```python
from build123d import *

# Parameters (mm, degrees)
SKETCH1_R           = 3.175
BOSS_EXTRUDE1_DEPTH = 3.175
SKETCH2_R           = 3.2004
SKETCH2_R_2         = 2.4384
SKETCH2_R_3         = 3.175
CUT_EXTRUDE2_DEPTH  = 205.115710138
SKETCH3_R           = 4.73075
CUT_EXTRUDE3_DEPTH  = 1.5875
CUT_EXTRUDE4_DEPTH  = 205.115710138


with BuildPart() as part:
    # Sketch1 → Boss-Extrude1 (new body)
    with BuildSketch(Plane(origin=(0, 0, 0), x_dir=(0, 0, -1), z_dir=(1, 0, 0))):
        with BuildLine():
            Line((12.7, 19.05), (0, 19.05))
            ThreePointArc((0, 19.05), (-19.05, 0), (0, -19.05))
            Line((0, -19.05), (12.7, -19.05))
            Line((12.7, -19.05), (12.7, -15.875))
            Line((12.7, -15.875), (25.4, -15.875))
            Line((25.4, -15.875), (25.4, -19.05))
            Line((25.4, -19.05), (38.1, -19.05))
            Line((38.1, -19.05), (38.1, -15.875))
            Line((38.1, -15.875), (50.8, -15.875))
            Line((50.8, -15.875), (50.8, -19.05))
            Line((50.8, -19.05), (63.5, -19.05))
            Line((63.5, -19.05), (63.5, -15.875))
            Line((63.5, -15.875), (76.2, -15.875))
            Line((76.2, -15.875), (76.2, -19.05))
            Line((76.2, -19.05), (88.9, -19.05))
            Line((88.9, -19.05), (88.9, -15.875))
            Line((88.9, -15.875), (101.6, -15.875))
            Line((101.6, -15.875), (101.6, -19.05))
            Line((101.6, -19.05), (114.3, -19.05))
            Line((114.3, -19.05), (114.3, -15.875))
            Line((114.3, -15.875), (127, -15.875))
            Line((127, -15.875), (127, -19.05))
            Line((127, -19.05), (139.7, -19.05))
            Line((139.7, -19.05), (139.7, -15.875))
            Line((139.7, -15.875), (152.4, -15.875))
            Line((152.4, -15.875), (152.4, -19.05))
            Line((152.4, -19.05), (165.1, -19.05))
            Line((165.1, -19.05), (165.1, -15.875))
            Line((165.1, -15.875), (177.8, -15.875))
            Line((177.8, -15.875), (177.8, -19.05))
            Line((177.8, -19.05), (190.5, -19.05))
            Line((190.5, -19.05), (190.5, -15.875))
            Line((190.5, -15.875), (203.2, -15.875))
            Line((203.2, -15.875), (203.2, 15.875))
            Line((203.2, 15.875), (190.5, 15.875))
            Line((190.5, 15.875), (190.5, 19.05))
            Line((190.5, 19.05), (177.8, 19.05))
            Line((177.8, 19.05), (177.8, 15.875))
            Line((177.8, 15.875), (165.1, 15.875))
            Line((165.1, 15.875), (165.1, 19.05))
            Line((165.1, 19.05), (152.4, 19.05))
            Line((152.4, 19.05), (152.4, 15.875))
            Line((152.4, 15.875), (139.7, 15.875))
            Line((139.7, 15.875), (139.7, 19.05))
            Line((139.7, 19.05), (127, 19.05))
            Line((127, 19.05), (127, 15.875))
            Line((127, 15.875), (114.3, 15.875))
            Line((114.3, 15.875), (114.3, 19.05))
            Line((114.3, 19.05), (101.6, 19.05))
            Line((101.6, 19.05), (101.6, 15.875))
            Line((101.6, 15.875), (88.9, 15.875))
            Line((88.9, 15.875), (88.9, 19.05))
            Line((88.9, 19.05), (76.2, 19.05))
            Line((76.2, 19.05), (76.2, 15.875))
            Line((76.2, 15.875), (63.5, 15.875))
            Line((63.5, 15.875), (63.5, 19.05))
            Line((63.5, 19.05), (50.8, 19.05))
            Line((50.8, 19.05), (50.8, 15.875))
            Line((50.8, 15.875), (38.1, 15.875))
            Line((38.1, 15.875), (38.1, 19.05))
            Line((38.1, 19.05), (25.4, 19.05))
            Line((25.4, 19.05), (25.4, 15.875))
            Line((25.4, 15.875), (12.7, 15.875))
            Line((12.7, 15.875), (12.7, 19.05))
        make_face()
        Circle(SKETCH1_R, mode=Mode.SUBTRACT)
    extrude(amount=BOSS_EXTRUDE1_DEPTH)

    # Sketch2 → Cut-Extrude2 (cut, through all)
    with BuildSketch(Plane(origin=(3.175, 0, 0), x_dir=(0, 0, -1), z_dir=(1, 0, 0))):
        with Locations((15.875, 0)):
            Circle(SKETCH2_R)
        with Locations((187.325, 0)):
            Circle(SKETCH2_R_2)
        with Locations((42.8625, 0)):
            Circle(SKETCH2_R_3)
        with Locations((77.7875, 0)):
            Circle(SKETCH2_R_3)
    extrude(amount=-CUT_EXTRUDE2_DEPTH, mode=Mode.SUBTRACT)

    # Sketch3 → Cut-Extrude3 (cut)
    with BuildSketch(Plane(origin=(3.175, 0, 0), x_dir=(0, 0, -1), z_dir=(1, 0, 0))):
        with Locations((15.875, 0)):
            Circle(SKETCH3_R)
        Polygon((3.229899478, -5.59435), (6.459798957, 0), (3.229899478, 5.59435), (-3.229899478, 5.59435), (-6.459798957, 0), (-3.229899478, -5.59435), align=None)
    extrude(amount=-CUT_EXTRUDE3_DEPTH, mode=Mode.SUBTRACT)

    # Sketch4 → Cut-Extrude4 (cut, through all)
    with BuildSketch(Plane(origin=(3.175, 0, 0), x_dir=(0, 0, -1), z_dir=(1, 0, 0))):
        with BuildLine():
            Line((133.35, 3.175), (158.75, 3.175))
            ThreePointArc((158.75, 3.175), (161.925, 0), (158.75, -3.175))
            Line((158.75, -3.175), (133.35, -3.175))
            ThreePointArc((133.35, -3.175), (130.175, 0), (133.35, 3.175))
        make_face()
    extrude(amount=-CUT_EXTRUDE4_DEPTH, mode=Mode.SUBTRACT)


solid = part.part
```
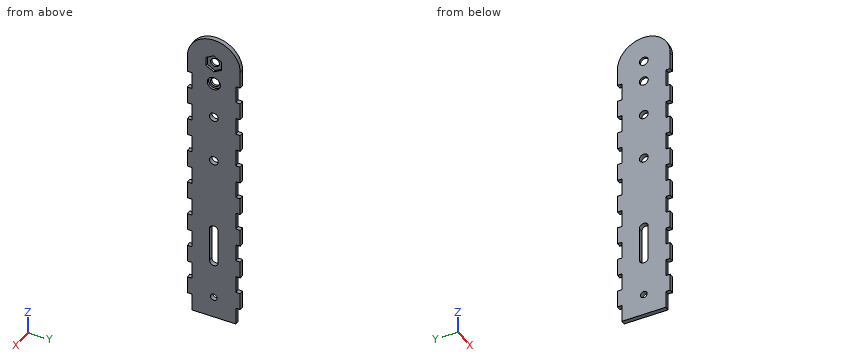
CAD build for the part. Positions are in the model's coordinates, mm. Coordinates: 2 decimals unless noted, no trailing zeros.
(1) Drill centre lines: L1, parallel to Z at x = 2.7, y = 2.5; L2, parallel to Y at x = 1.8, z = -50 (3 decimals); L3, parallel to Y at x = 0.4, z = -2. Where is each one in solid material? Low to high.
Solution:
L1: z = -203.2 to -160.71, -131.39 to -79.74, -75.83 to -44.82, -40.91 to -19.89, -11.86 to -5.02, 5.02 to 18.89
L2: y = -15.875 to 15.875
L3: y = -19.05 to -2.47, 2.47 to 19.05
(2) Saw through at A-A, the plane x = 0.7. Count the separate pieces of the cut face and the enclosed holes in it, and give its area (3 significant figures).
Solution:
separate pieces: 1
enclosed holes: 6
area: 7,330 mm2
(3) Pin check, flat tips, straight feed: pin 1 Ø1.6 at (x, z) = (1.5, -142) entering from +Y (3 decimals); pin 2 Ø4.5 at (y, z) = (0.5, -15) entering from +X; pin 3 Ø1 at (x, z) = (1, -21) entering from -Y (3 decimals). Stop position of each tip, or through.
Solution:
pin 1: stops at y = 15.875
pin 2: stops at x = 1.59
pin 3: stops at y = -15.875
